```python
from build123d import *

# Parameters (mm, degrees)
SKETCH2_W           = 150
SKETCH2_H           = 200
BOSS_EXTRUDE1_DEPTH = 30
SKETCH3_R           = 10
CUT_EXTRUDE1_DEPTH  = 30
SKETCH4_R           = 15
CUT_EXTRUDE2_DEPTH  = 15
SKETCH6_R           = 7.5
CUT_EXTRUDE3_DEPTH  = 30
SKETCH7_R           = 4.5
CUT_EXTRUDE4_DEPTH  = 30
SKETCH9_R           = 6.25
CUT_EXTRUDE6_DEPTH  = 9


with BuildPart() as part:
    # Sketch2 → Boss-Extrude1 (new body)
    with BuildSketch(Plane(origin=(0, 0, 0), x_dir=(0, 0, -1), z_dir=(1, 0, 0))):
        with Locations((-75, 100)):
            Rectangle(SKETCH2_W, SKETCH2_H)
    extrude(amount=BOSS_EXTRUDE1_DEPTH)

    # Sketch3 → Cut-Extrude1 (cut)
    with BuildSketch(Plane(origin=(30, 0, 0), x_dir=(0, 0, -1), z_dir=(1, 0, 0))):
        with Locations((-112.5, 175)):
            Circle(SKETCH3_R)
        with Locations(Location((-37.5, 175, 0), (0, 0, 180))):
            Circle(SKETCH3_R)
        with Locations((-112.5, 135)):
            Circle(SKETCH3_R)
        with Locations(Location((-37.5, 135, 0), (0, 0, 180))):
            Circle(SKETCH3_R)
    extrude(amount=-CUT_EXTRUDE1_DEPTH, mode=Mode.SUBTRACT)

    # Sketch4 → Cut-Extrude2 (cut)
    with BuildSketch(Plane(origin=(30, 0, 0), x_dir=(0, 0, -1), z_dir=(1, 0, 0))):
        with Locations((-75, 50)):
            Circle(SKETCH4_R)
    extrude(amount=-CUT_EXTRUDE2_DEPTH, mode=Mode.SUBTRACT)

    # Sketch6 → Cut-Extrude3 (cut)
    with BuildSketch(Plane(origin=(30, 0, 0), x_dir=(0, 0, -1), z_dir=(1, 0, 0))):
        with Locations((-75, 50)):
            Circle(SKETCH6_R)
    extrude(amount=-CUT_EXTRUDE3_DEPTH, mode=Mode.SUBTRACT)

    # Sketch7 → Cut-Extrude4 (cut)
    with BuildSketch(Plane(origin=(30, 0, 0), x_dir=(0, 0, -1), z_dir=(1, 0, 0))):
        with Locations((-125, 50)):
            Circle(SKETCH7_R)
        with Locations((-25, 50)):
            Circle(SKETCH7_R)
    extrude(amount=-CUT_EXTRUDE4_DEPTH, mode=Mode.SUBTRACT)

    # Sketch9 → Cut-Extrude6 (cut)
    with BuildSketch(Plane(origin=(30, 0, 0), x_dir=(0, 0, -1), z_dir=(1, 0, 0))):
        with Locations((-125, 50)):
            Circle(SKETCH9_R)
        with Locations((-25, 50)):
            Circle(SKETCH9_R)
    extrude(amount=-CUT_EXTRUDE6_DEPTH, mode=Mode.SUBTRACT)


solid = part.part
```
Here's how the part is built. I have some questions about the finished solid (model axes, mm). A direction names the side the tool comes from. Coordinates: 2 decimals unless noted, no trailing zeros. Order: outer loops, then holes, each group sorted by start corner. A loop starts at its lowest first (then second) coordinate and runs counter-clockwise, first axis right, second up.
1) Imagine slicing it at B-B on x = 24. List the corners of the cut face in (y, z) for me.
2) I need wall thicknesses on line 1 (Y direction, x = 18.25, z = 112.5); line 2 (Z direction, x = 18.5, y = 181); line 3 (Y direction, x = 4.75, z = 115.5). Which ranges of each line are inside material? Lowest first, please.
3) Imagine slicing it at A-A on y = 175. List the corners of the cut face in (x, z) for me, and give its area (3 significant figures).
4) Imagine slicing it at D-D on y = 50. List the corners of the cut face in (x, z) for me, and give its area (3 significant figures).
5) We'd pull the mould along Z, two halves only. Please class faces 3 (the face through (15.21, 165.24, 114.67)), 4 (the face through (15, 99, 0)), 5 (the face through (22.605, 64.872, 76.953)), 6 (the face through (15, 0, 76)): +Z half, -Z half, draft (parallel to the pull), parting line (faces both ways), or undercut.
6) Which directions (+Z, -Z, +X, -X, +Y, -Y) give clear straight access to the entire face, cutting with the end or side of a thin tool? Please do faces 1 (the face through (15, 57, 79)), 2 (the face through (0, 101, 76)).
7) Will these pins go through, and if not, where does the flat tip stop? pin 1 (10 mm diameter, centred on y = 50, z = 125, fed in from +X); pin 2 (15 mm diameter, centred on y = 46.5, z = 72, fed in from +X).
8) Imagine slicing it at C-C on z = 112.5. List the corners of the cut face in (x, y) for me, and give its area (3 significant figures).
Response values:
1. outline: (0, 0) - (200, 0) - (200, 150) - (0, 150) - close; hole circle Ø30 at (50, 75); hole circle Ø12.5 at (50, 25); hole circle Ø12.5 at (50, 125); hole circle Ø20 at (135, 37.5); hole circle Ø20 at (135, 112.5); hole circle Ø20 at (175, 37.5); hole circle Ø20 at (175, 112.5)
2. line 1: y = 0 to 125, 145 to 165, 185 to 200
2. line 2: z = 0 to 29.5, 45.5 to 104.5, 120.5 to 150
2. line 3: y = 0 to 125.46, 144.54 to 165.46, 184.54 to 200
3. outline: (0, 0) - (30, 0) - (30, 27.5) - (0, 27.5) - close; (0, 47.5) - (30, 47.5) - (30, 102.5) - (0, 102.5) - close; (0, 122.5) - (30, 122.5) - (30, 150) - (0, 150) - close
3. area: 3,300 mm2
4. outline: (0, 0) - (30, 0) - (30, 18.75) - (21, 18.75) - (21, 20.5) - (0, 20.5) - close; (0, 29.5) - (21, 29.5) - (21, 31.25) - (30, 31.25) - (30, 60) - (15, 60) - (15, 67.5) - (0, 67.5) - close; (0, 82.5) - (15, 82.5) - (15, 90) - (30, 90) - (30, 118.75) - (21, 118.75) - (21, 120.5) - (0, 120.5) - close; (0, 129.5) - (21, 129.5) - (21, 131.25) - (30, 131.25) - (30, 150) - (0, 150) - close
4. area: 3,220 mm2
5. face 3: undercut
5. face 4: -Z half
5. face 5: undercut
5. face 6: draft
6. face 1: +X
6. face 2: +Z, -Z, -X, +Y, -Y
7. pin 1: stops at x = 21
7. pin 2: stops at x = 15
8. outline: (0, 0) - (30, 0) - (30, 125) - (0, 125) - close; (0, 145) - (30, 145) - (30, 165) - (0, 165) - close; (0, 185) - (30, 185) - (30, 200) - (0, 200) - close
8. area: 4,800 mm2
